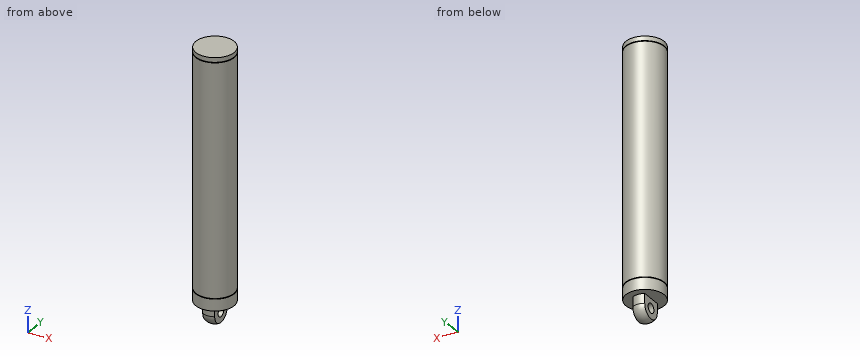
Autodesk Inventor part; units mm, degrees
ref_plane "BodyCapPlane" through (0, 0, 101.5) normal (0, 0, 1) x (1, 0, 0)
ref_plane "BaseBodyPlane" through (0, 0, 5) normal (0, 0, 1) x (1, 0, 0)
ref_plane "YZ Plane" through (0, 0, 0) normal (1, 0, 0) x (0, 1, 0)
sketch "Base" plane through (0, 0, 0) normal (0, 0, 1) x (1, 0, 0)
  circle A0 centre (0, 0) radius 8
  dimension "d0" = 16
extrude "BaseFeature" add sketch "Base" along normal blind 5
sketch "Mount" plane through (0, 0, 0) normal (0, 0, -1) x (-1, 0, 0)
  line L0 (2.5, -5) -> (-2.5, -5)
  line L1 (-2.5, -5) -> (-2.5, 5)
  line L2 (-2.5, 5) -> (2.5, 5)
  line L3 (2.5, 5) -> (2.5, -5)
  line L4 (11.2, 0) -> (-11.2, 0) construction
  line L5 (0, -11.2) -> (0, 11.2) construction
  circle A0 centre (0, 0) radius 5
  point P0 (0, -5)
  point P1 (2.5, 4.3301)
  point P2 (-2.5, 4.3301)
  point P3 (-2.5, -4.3301)
  point P4 (2.5, -4.3301)
  dimension "d3" = 10
  dimension "d4" = 5
extrude "MountFeature" add sketch "Mount" along normal blind 9 contours A0 L1 L3
sketch "MountProfile" plane through (0, 0, 0) normal (1, 0, 0) x (0, 1, 0)
  line L0 (5, 0) -> (5, -9)
  line L1 (4.3301, -9) -> (5, -9)
  line L2 (4.3301, -9) -> (-4.3301, -9)
  line L3 (-5, -9) -> (-4.3301, -9)
  line L4 (-5, 0) -> (-5, -9)
  line L5 (8, 0) -> (-8, 0)
  circle A0 centre (0, -4) radius 5
  line L6 (5, -4) -> (-5, -4)
  line L7 (0, -11) -> (0, 3)
  point P0 (0, 0)
  point P1 (0, -4)
  point P2 (0, -9)
  point P3 (-5, -4)
  point P4 (5, -4)
revolve "MountProfileFeature" cut sketch "MountProfile" angle 360 about axis through (0, 0, -10) along (0, 0, 1) contours L0 L1 L2 A0 | L2 L3 L4 A0
sketch "MountHole" plane through (2.5, -4.3301, 0) normal (1, 0, 0) x (0, 0, -1)
  arc A0 (4, 0) -> (4, 8.6603) centre (4, 4.3301) ccw
  circle A1 centre (4, 4.3301) radius 2
  point P0 (0, 4.3301)
  dimension "d15" = 4
extrude "MountHoleFeature" cut sketch "MountHole" against normal blind 10
sketch "Body" plane through (0, 0, 5) normal (0, 0, 1) x (1, 0, 0)
  circle A0 centre (0, 0) radius 8
extrude "BodyFeature" add sketch "Body" along normal blind 96.5
ref_plane "BodyCapPlane" through (0, 0, 101.5) normal (0, 0, 1) x (1, 0, 0)
ref_plane "BaseBodyPlane" through (0, 0, 5) normal (0, 0, 1) x (1, 0, 0)
sketch "Sketch9" plane through (0, 0, 101.5) normal (0, 0, 1) x (1, 0, 0)
  circle A0 centre (0, 0) radius 8
extrude "BodyCapFeature" add sketch "Sketch9" along normal blind 2
sketch "BodyCapEtch" plane through (0, 0, 101.5) normal (0, 0, 1) x (1, 0, 0)
  circle A0 centre (0, 0) radius 8
  circle A1 centre (0, 0) radius 7.75
  dimension "d24" = 0.25
extrude "BodyCapEtchFeature" cut sketch "BodyCapEtch" along normal mid plane 0.25
sketch "BodyBaseEtch" plane through (0, 0, 5) normal (0, 0, 1) x (1, 0, 0)
  circle A0 centre (0, 0) radius 8
  circle A1 centre (0, 0) radius 7.75
  dimension "d27" = 0.25
extrude "BodyBaseEtchFeature" cut sketch "BodyBaseEtch" along normal mid plane 0.25
properties part number "1610-50H-2KG-12V-B07-Body"
Part model, mm, in its own coordinate system. Round coordinates to 2 decimals unless told otherwise and drop trailing zeros. Loops run counter-clockwise (first coordinate to the right, second up) from the corner with the lowest first, then second, coordinate; pieces in that order, holes last.
Item 1: Drop flat-ended pins along their axis: P1, Ø5, axis at x = -3, y = -1.5, coming from the -Z side; P2, Ø8, axis at x = -4.5, z = 38.5, coming from the -Y side; P3, Ø6, axis at x = 4, z = 14, coming from the -Y side; P4, Ø3, axis at y = 0, z = -4, coming from the +X side. Give the stop position or say it passes through.
Item 2: Cut at B-B, the plane x = 0. Give the cut face in (y, z) (3 decimals), then the cut area to 3 significant figures.
Item 3: Cut at D-D, the plane x = 4.25. Give the cut face in (y, z) (3 decimals), then the cut area to 3 significant figures.
Item 4: Drill centre lines: line 1 (Z direction, x = 4, y = 6.75) (3 decimals); line 2 (Y direction, x = -0.15, z = -4); line 3 (Z direction, x = -3.75, y = -6.75). Where is each one in solid material? Low to high.
Item 5: Cut at A-A, the plane y = 0. Give the cut face in (x, z) (3 decimals), then the cut area to 3 significant figures.
Item 6: Cut at C-C, the plane z = 7.5. Give the cut face in (x, y), then the cut area to 3 significant figures.
A:
1. P1: stops at z = -8.93
1. P2: stops at y = -7.98
1. P3: stops at y = -7.94
1. P4: passes through
2. outline: (-8, 0) - (-5, 0) - (-5, -4) arc R5 ccw to (5, -4) - (5, 0) - (8, 0) - (8, 4.875) - (7.75, 4.875) - (7.75, 5.125) - (8, 5.125) - (8, 101.375) - (7.75, 101.375) - (7.75, 101.625) - (8, 101.625) - (8, 103.5) - (-8, 103.5) - (-8, 101.625) - (-7.75, 101.625) - (-7.75, 101.375) - (-8, 101.375) - (-8, 5.125) - (-7.75, 5.125) - (-7.75, 4.875) - (-8, 4.875) - close; hole circle Ø4 at (0, -4)
2. area: 1,720 mm2
3. outline: (-6.778, 0) - (6.778, 0) - (6.778, 4.875) - (6.481, 4.875) - (6.481, 5.125) - (6.778, 5.125) - (6.778, 101.375) - (6.481, 101.375) - (6.481, 101.625) - (6.778, 101.625) - (6.778, 103.5) - (-6.778, 103.5) - (-6.778, 101.625) - (-6.481, 101.625) - (-6.481, 101.375) - (-6.778, 101.375) - (-6.778, 5.125) - (-6.481, 5.125) - (-6.481, 4.875) - (-6.778, 4.875) - close
3. area: 1,400 mm2
4. line 1: z = 0 to 4.875, 5.125 to 101.375, 101.625 to 103.5
4. line 2: y = -5 to -2, 2 to 5
4. line 3: z = 0 to 103.5
5. outline: (-8, 0) - (-2.5, 0) - (-2.5, -2) - (2.5, -2) - (2.5, 0) - (8, 0) - (8, 4.875) - (7.75, 4.875) - (7.75, 5.125) - (8, 5.125) - (8, 101.375) - (7.75, 101.375) - (7.75, 101.625) - (8, 101.625) - (8, 103.5) - (-8, 103.5) - (-8, 101.625) - (-7.75, 101.625) - (-7.75, 101.375) - (-8, 101.375) - (-8, 5.125) - (-7.75, 5.125) - (-7.75, 4.875) - (-8, 4.875) - close; (-2.5, -8.33) arc R5 ccw to (2.5, -8.33) - (2.5, -6) - (-2.5, -6) - close
5. area: 1,680 mm2
6. outline: circle Ø16 at (0, 0)
6. area: 201 mm2
